from build123d import *

# Parameters (mm, degrees)
BOSS_EXTRUDE1_DEPTH          = 10
CONVERT_SOLID1_DEPTH         = 6
EDGE_FLANGE2_DEPTH           = 600
EDGE_FLANGE4_STRIP_CUT_DEPTH = 600
EDGE_FLANGE4_DEPTH           = 600
CUT_EXTRUDE2_DEPTH           = 952.374861111
CUT_EXTRUDE2_DEPTH_BACK      = 952.374861111
TAB1_DEPTH                   = 4


# Read off the part's stored shape, not the designer's step: Convert-Solid1
# Sheet-metal steps are written as plain solids
with BuildPart() as part:
    # Sketch1 → Boss-Extrude1 (new body)
    with BuildSketch(Plane(origin=(0, 0, 0), x_dir=(1, 0, 0), z_dir=(0, 1, 0))):
        Polygon((-192.279765905, 237.5), (404.456147209, 300), (404.456147209, 0), (404.456147209, -300), (-192.279765905, -237.5), align=None)
    extrude(amount=BOSS_EXTRUDE1_DEPTH)

    # Convert-Solid1 outline → Convert-Solid1 (cut)
    with BuildSketch(Plane(origin=(0, 0, 0), x_dir=(1, 0, 0), z_dir=(0, 1, 0))):
        Polygon((-192.279765905, 237.5), (-192.279765905, -237.5), (404.456147209, -300), (404.456147209, 300), align=None)
    extrude(amount=CONVERT_SOLID1_DEPTH, mode=Mode.SUBTRACT)

    # Edge-Flange2 section (across the edge) → Edge-Flange2 (add)
    with BuildSketch(Plane(origin=(414.456147209, 10, 300), x_dir=(-0.9659258262890673, 0.25881904510252446, 0), z_dir=(0, 0, -1))):
        with BuildLine():
            Line((-4, 7.67326988), (-4, 187.930692048))
            Line((-4, 187.930692048), (0, 187.930692048))
            Line((0, 187.930692048), (0, 7.67326988))
            ThreePointArc((0, 7.67326988), (2.066466597, 1.58565559), (7.411809549, -1.985988383))
            Line((7.411809549, -1.985988383), (9.659258263, -2.588190451))
            Line((9.659258263, -2.588190451), (8.623982082, -6.451893756))
            Line((8.623982082, -6.451893756), (6.376533369, -5.849691688))
            ThreePointArc((6.376533369, -5.849691688), (-1.106946764, -0.849390126), (-4, 7.67326988))
        make_face()
    extrude(amount=EDGE_FLANGE2_DEPTH)

    # Edge-Flange4 strip (across the edge) → Edge-Flange4 strip cut (cut)
    with BuildSketch(Plane(origin=(463.09618947, 191.527109002, 300), x_dir=(-0.9961946980917449, 0.0871557427476667, 0), z_dir=(0, 0, -1))):
        Polygon((-10.038642938, 33.896891256), (-3.787308542, -1.556187852), (0.15192247, -0.861595141), (-6.099411926, 34.591483967), align=None)
    extrude(amount=EDGE_FLANGE4_STRIP_CUT_DEPTH, mode=Mode.SUBTRACT)

    # Edge-Flange4 section (across the edge) → Edge-Flange4 (add)
    with BuildSketch(Plane(origin=(463.09618947, 191.527109002, 300), x_dir=(-0.9961946980917449, 0.0871557427476667, 0), z_dir=(0, 0, -1))):
        with BuildLine():
            Line((-4, 0.874886635), (-4, 412.850045346))
            Line((-4, 412.850045346), (0, 412.850045346))
            Line((0, 412.850045346), (0, 0.874886635))
            ThreePointArc((0, 0.874886635), (0.038053019, 0.003329208), (0.15192247, -0.861595141))
            Line((0.15192247, -0.861595141), (-3.787308542, -1.556187852))
            ThreePointArc((-3.787308542, -1.556187852), (-3.946725773, -0.345293763), (-4, 0.874886635))
        make_face()
    extrude(amount=EDGE_FLANGE4_DEPTH)

    # Sketch22 → Cut-Extrude2 (cut, two sides: drawn at the far end of the back side and taken through both)
    with BuildSketch(Plane(origin=(442.9492869, -38.753041121, 0), x_dir=(0, 0, 1), z_dir=(-0.9961946980917449, 0.08715574274766662, 0)).offset(-CUT_EXTRUDE2_DEPTH_BACK)):
        Polygon((300, 232.03466952), (196.591479546, 525.272945681), (153.798650158, 525.272945681), (87.551647761, 644.009828231), (302.699803465, 645.121208779), (304.833664863, 232.03466952), align=None)
        Polygon((-300, 232.03466952), (-196.591479546, 525.272945681), (-153.798650158, 525.272945681), (-87.551647761, 644.009828231), (-302.699803465, 645.121208779), (-304.833664863, 232.03466952), align=None)
    extrude(amount=CUT_EXTRUDE2_DEPTH + CUT_EXTRUDE2_DEPTH_BACK, mode=Mode.SUBTRACT)

    # Sketch24 → Tab1 (add)
    with BuildSketch(Plane(origin=(0, 10, 0), x_dir=(1, 0, 0), z_dir=(0, 1, 0))):
        Polygon((-192.279765905, 237.5), (-887.537085834, 187.5), (-887.537085834, -187.5), (-192.279765905, -237.5), align=None)
    extrude(amount=-TAB1_DEPTH)


solid = part.part
The model under review builds one solid part; all positions refer to its coordinate system, in mm. Coordinates: 2 decimals unless noted, no trailing zeros. Write each loop counter-clockwise with the first axis right and the second up, starting at its lowest first coordinate (ties: lowest second). Pieces come first, ordered by that corner, then holes. Notation, with made-up numbers: (42.5, -1) - (62.5, -1) arc R13 cw to (62.5, 18) - close; hole circle Ø11 at (51, 55.25). An arc over 180 degrees is marked (long way). Answer as a JSON object with one key per item and string values. Group by question number.
1. Clearance check with flat-ended pins moving along their axes: pin 1 Ø2 at (y, z) = (430, 33.5) entering from +X; pin 2 Ø1.5 at (x, z) = (-53.5, 222) entering from +Y; pin 3 Ø2 at (y, z) = (286.5, -228.5) entering from -X. State where each tip first meets the part, or that it passes through.
2. Add section B-B (x = -329). Give the boundary of the cut face in (y, z), plus the area to 3 significant figures.
3. To check wall thickness, follow probe 1 along Y at (x, z) = (-804, -43); probe 2 along X at (y, z) = (142, -9); probe 3 along X at (y, z) = (241, 141). State the ranges of each line that lie inside material, in increasing order.
4. Add section A-A (z = 134). Give the boundary of the cut face in (x, y).
5. Add section D-D (z = -254). Give the boundary of the cut face in (x, y), plus the area to 3 significant figures.
6. Add section C-C (y = 133). Give the boundary of the cut face in (x, z) (3 decimals), plus the area to 3 significant figures.
Findings:
{
 "1": {"pin 1": "x = 488.06", "pin 2": "y = 10", "pin 3": "x = 471.32"},
 "2": {"outline": "(6, -227.67) - (10, -227.67) - (10, 227.67) - (6, 227.67) - close", "area": "1,820 mm²"},
 "3": {"probe 1": "6 to 10", "probe 2": "449.83 to 453.97", "probe 3": "467.42 to 471.44"},
 "4": {"outline": "(-887.54, 6) - (406.78, 6) arc R14 ccw to (420.31, 16.38) - (466.73, 189.65) arc R14 ccw to (467.16, 192.05) - (495.81, 519.52) - (491.82, 519.87) - (463.17, 192.4) arc R10 cw to (462.87, 190.68) - (416.44, 17.41) arc R10 cw to (406.78, 10) - (-887.54, 10) - close"},
 "5": {"outline": "(-34.74, 6) - (406.78, 6) arc R14 ccw to (420.31, 16.38) - (466.73, 189.65) arc R14 ccw to (467.16, 192.05) - (478.53, 322) - (474.54, 322.35) - (463.17, 192.4) arc R10 cw to (462.87, 190.68) - (416.44, 17.41) arc R10 cw to (406.78, 10) - (-34.74, 10) - close", "area": "3,080 mm²"},
 "6": {"outline": "(447.414, -300) - (451.555, -300) - (451.555, 300) - (447.414, 300) - close", "area": "2,480 mm²"}
}
